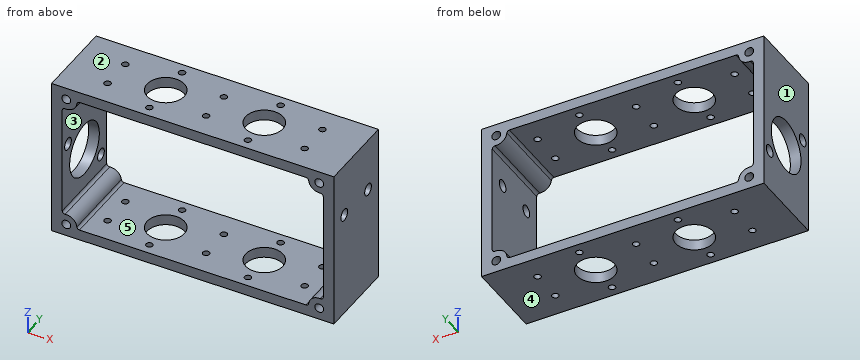
from build123d import *

# Parameters (mm, degrees)
SKETCH_1_W                                 = 106
SKETCH_1_H                                 = 60
EXTRUDE_1_DEPTH                            = 15
SKETCH_4_W                                 = 98
SKETCH_4_H                                 = 52
CUT_EXTRUDE_3_DEPTH                        = 68.88961629
SKETCH_5_R                                 = 2
EXTRUDE_2_DEPTH                            = 30
MIRROR_3_COPY_1_SKETCH_R                   = 2
MIRROR_3_COPY_1_DEPTH                      = 30
SKETCH_3_R                                 = 1.65
CUT_EXTRUDE_2_DEPTH                        = 10
CUT_EXTRUDE_4_REACH                        = 113.18
SKETCH_6_R                                 = 10
SKETCH_6_R_2                               = 2.25
SKETCH_7_R                                 = 2.25
CUT_EXTRUDE_5_DEPTH                        = 108.373181009
SKETCH_8_R                                 = 7
CUT_EXTRUDE_6_DEPTH                        = 82.449370777
HOLE_WIZARD_M3_1_D                         = 2.5
MIRROR_4_AT_THE_SECOND_PLANE_COPY_1_SKET_R = 7
MIRROR_4_AT_THE_SECOND_PLANE_COPY_1_DEPTH  = 82.449370777
MIRROR_4_AT_THE_SECOND_PLANE_COPY_2_D      = 2.5
EXTRUDE_START                              = -30
EXTRUDE_3_DEPTH                            = 30
FILLET_1_R                                 = 1


with BuildPart() as part:
    # 草图1 → 凸台-拉伸1 (new, symmetric)
    with BuildSketch(Plane(origin=(0, 0, 0), x_dir=(1, 0, 0), z_dir=(0, 1, 0))):
        Rectangle(SKETCH_1_W, SKETCH_1_H)
    extrude(amount=EXTRUDE_1_DEPTH, both=True)

    # 草图4 → 切除-拉伸3 (cut, through all)
    with BuildSketch(Plane(origin=(0, 15, 0), x_dir=(1, 0, 0), z_dir=(0, 1, 0))):
        Rectangle(SKETCH_4_W, SKETCH_4_H)
    extrude(amount=-CUT_EXTRUDE_3_DEPTH, mode=Mode.SUBTRACT)

    # 草图5 → 凸台-拉伸2 (add)
    with BuildSketch(Plane(origin=(0, 15, 0), x_dir=(1, 0, 0), z_dir=(0, 1, 0))):
        with Locations((47.5, 25.5)):
            Circle(SKETCH_5_R)
    extrude_2 = extrude(amount=-EXTRUDE_2_DEPTH)

    # 镜向2: 凸台-拉伸2 across plane
    add(extrude_2.mirror(Plane(origin=(0, 0, 0), x_dir=(0, 0, 1), z_dir=(1, 0, 0))))

    # 镜向3: 凸台-拉伸2 across plane
    add(extrude_2.mirror(Plane.XY))

    # 镜向3 copy 1 sketch → 镜向3 copy 1 (add)
    with BuildSketch(Plane(origin=(0, 15, 0), x_dir=(-1, 0, 0), z_dir=(0, 1, 0))):
        with Locations((47.5, 25.5)):
            Circle(MIRROR_3_COPY_1_SKETCH_R)
    extrude(amount=-MIRROR_3_COPY_1_DEPTH)

    # 草图3 → 切除-拉伸2 (cut)
    with BuildSketch(Plane(origin=(0, 15, 0), x_dir=(1, 0, 0), z_dir=(0, 1, 0))):
        with Locations(Location((47.5, 25.5, 0), (0, 0, 270))):
            Circle(SKETCH_3_R)
        with Locations(Location((47.5, -25.5, 0), (0, 0, 90))):
            Circle(SKETCH_3_R)
        with Locations(Location((-47.5, -25.5, 0), (0, 0, 270))):
            Circle(SKETCH_3_R)
        with Locations(Location((-47.5, 25.5, 0), (0, 0, 90))):
            Circle(SKETCH_3_R)
    cut_extrude_2 = extrude(amount=-CUT_EXTRUDE_2_DEPTH, mode=Mode.SUBTRACT)

    # 镜向1: 切除-拉伸2 across plane
    add(cut_extrude_2.mirror(Plane.ZX), mode=Mode.SUBTRACT)

    # 草图6 → 切除-拉伸4 (cut, up to next)
    with BuildSketch(Plane.ZY.offset(53), mode=Mode.PRIVATE) as cut_extrude_4_sk1:
        with Locations((-5, 0)):
            Circle(SKETCH_6_R)
    cut_extrude_4_tool1 = extrude(cut_extrude_4_sk1.sketch, amount=-CUT_EXTRUDE_4_REACH, mode=Mode.PRIVATE) & part.part
    # 草图6 → 切除-拉伸4 (cut, up to next)
    with BuildSketch(Plane.ZY.offset(53), mode=Mode.PRIVATE) as cut_extrude_4_sk2:
        with Locations((-14.32042034, 11.107644425)):
            Circle(SKETCH_6_R_2)
    cut_extrude_4_tool2 = extrude(cut_extrude_4_sk2.sketch, amount=-CUT_EXTRUDE_4_REACH, mode=Mode.PRIVATE) & part.part
    # 草图6 → 切除-拉伸4 (cut, up to next)
    with BuildSketch(Plane.ZY.offset(53), mode=Mode.PRIVATE) as cut_extrude_4_sk3:
        with Locations((4.32042034, -11.107644425)):
            Circle(SKETCH_6_R_2)
    cut_extrude_4_tool3 = extrude(cut_extrude_4_sk3.sketch, amount=-CUT_EXTRUDE_4_REACH, mode=Mode.PRIVATE) & part.part
    add(cut_extrude_4_tool1.solids().sort_by_distance((-53, 0, -5))[0], mode=Mode.SUBTRACT)
    add(cut_extrude_4_tool2.solids().sort_by_distance((-53, 11.107644, -14.32042))[0], mode=Mode.SUBTRACT)
    add(cut_extrude_4_tool3.solids().sort_by_distance((-53, -11.107644, 4.32042))[0], mode=Mode.SUBTRACT)

    # 草图7 → 切除-拉伸5 (cut, through all)
    with BuildSketch(Plane.ZY.offset(-49)):
        with Locations((10, 8)):
            Circle(SKETCH_7_R)
        with Locations((10, -8)):
            Circle(SKETCH_7_R)
    extrude(amount=-CUT_EXTRUDE_5_DEPTH, mode=Mode.SUBTRACT)

    # 草图8 → 切除-拉伸6 (cut, through all)
    with BuildSketch(Plane.XY.offset(30)):
        with Locations((18.5, 0)):
            Circle(SKETCH_8_R)
    cut_extrude_6 = extrude(amount=-CUT_EXTRUDE_6_DEPTH, mode=Mode.SUBTRACT)

    # M3 螺纹孔1 (through all)
    with Locations(Plane(origin=(0, 6, 30), x_dir=(1, 0, 0), z_dir=(0, 0, 1))):
        with Locations((0, 0), (18.5, 5), (37, 0)):
            hole_wizard_m3_1 = Hole(HOLE_WIZARD_M3_1_D / 2)

    # 镜向4: 切除-拉伸6, M3 螺纹孔1 across plane
    add(cut_extrude_6.mirror(Plane(origin=(0, 0, 0), x_dir=(0, 0, 1), z_dir=(1, 0, 0))), mode=Mode.SUBTRACT)
    add(hole_wizard_m3_1.mirror(Plane(origin=(0, 0, 0), x_dir=(0, 0, 1), z_dir=(1, 0, 0))), mode=Mode.SUBTRACT)

    # 镜向4 at the second plane: 切除-拉伸6, M3 螺纹孔1 across plane
    add(cut_extrude_6.mirror(Plane.ZX), mode=Mode.SUBTRACT)
    add(hole_wizard_m3_1.mirror(Plane.ZX), mode=Mode.SUBTRACT)

    # 镜向4 at the second plane copy 1 sket → 镜向4 at the second plane copy 1 (cut, through all)
    with BuildSketch(Plane(origin=(0, 0, 30), x_dir=(-1, 0, 0), z_dir=(0, 0, 1))):
        with Locations((18.5, 0)):
            Circle(MIRROR_4_AT_THE_SECOND_PLANE_COPY_1_SKET_R)
    extrude(amount=-MIRROR_4_AT_THE_SECOND_PLANE_COPY_1_DEPTH, mode=Mode.SUBTRACT)

    # 镜向4 at the second plane copy 2 (through all)
    with Locations(Plane(origin=(0, -6, 30), x_dir=(-1, 0, 0), z_dir=(0, 0, 1))):
        with Locations((0, 0), (18.5, 5), (37, 0)):
            Hole(MIRROR_4_AT_THE_SECOND_PLANE_COPY_2_D / 2)

    # 草图10 → 凸台-拉伸3 (add)
    with BuildSketch(Plane(origin=(0, 15, 0), x_dir=(1, 0, 0), z_dir=(0, 1, 0)).offset(EXTRUDE_START)):
        with BuildLine():
            ThreePointArc((-49, 21.791900756), (-45.06062414, 22.329913974), (-43.531373033, 26))
            Line((-43.531373033, 26), (-45.563508327, 26))
            ThreePointArc((-45.563508327, 26), (-46.562796629, 23.733180869), (-49, 24.177124344))
            Line((-49, 24.177124344), (-49, 21.791900756))
        make_face()
        with BuildLine():
            Line((45.563508327, 26), (43.531373033, 26))
            ThreePointArc((43.531373033, 26), (45.06062414, 22.329913974), (49, 21.791900756))
            Line((49, 21.791900756), (49, 24.177124344))
            ThreePointArc((49, 24.177124344), (46.562796629, 23.733180869), (45.563508327, 26))
        make_face()
        with BuildLine():
            ThreePointArc((-43.531373033, -26), (-45.06062414, -22.329913974), (-49, -21.791900756))
            Line((-49, -21.791900756), (-49, -24.177124344))
            ThreePointArc((-49, -24.177124344), (-46.562796629, -23.733180869), (-45.563508327, -26))
            Line((-45.563508327, -26), (-43.531373033, -26))
        make_face()
        with BuildLine():
            Line((49, -24.177124344), (49, -21.791900756))
            ThreePointArc((49, -21.791900756), (45.06062414, -22.329913974), (43.531373033, -26))
            Line((43.531373033, -26), (45.563508327, -26))
            ThreePointArc((45.563508327, -26), (46.562796629, -23.733180869), (49, -24.177124344))
        make_face()
    extrude(amount=EXTRUDE_3_DEPTH)

    # 圆角1
    fillet_1_edges = [part.edges().sort_by_distance(p)[0] for p in [
        (49, 0, -21.791900756),
        (43.531373033, 0, -26),
        (43.531373033, 0, 26),
        (49, 0, 21.791900756),
        (-49, 0, 21.791900756),
        (-43.531373033, 0, 26),
        (-43.531373033, 0, -26),
        (-49, 0, -21.791900756),
    ]]
    fillet(fillet_1_edges, radius=FILLET_1_R)


solid = part.part
Source: CAD feature listing. Evaluate the final solid. Frame: model axes, mm. Face numbers are marked on the shaded views. A direction names the side the tool comes from. Give positions to 0.01 mm unless a question says otherwise; leave off trailing zeros. Write each loop counter-clockwise with the first axis right and the second up, starting at its lowest first coordinate (ties: lowest second). Pieces come first, ordered by that corner, then holes. Notation, with made-up numbers: (0, 52) - (22, 52) arc R20 ccw to (22, 85) - close; hole circle Ø3 at (-29, 1.25). An arc over 180 degrees is marked (long way). Write item = value, one per line. Start each with the question number.
Q1. Cut plane A-A, the plane x = 8. Return loops of the section in (y, z), then the cut area to 3 significant figures.
Q2. Draft query along X for the marked faces 1, 2 and 3. Return one class per face: +X half, -X half, draft (parallel to the pull), parting line (faces both ways), or undercut.
Q3. Pin query (flat end, axial travel): pin 1 Ø5 at (y, z) = (0.5, 1) entering from -X; pin 2 Ø2 at (x, z) = (-47.5, 25.5) entering from -Y. Return the tip coordinate at first contact, or that it passes through.
Q4. Material intervals for probe 1 along Y at (x, z) = (0, -28.35); probe 2 along Y at (x, z) = (-18.5, -28.4); probe 3 along Y at (x, z) = (51.25, 10), sorted ascending.
Q5. Cut plane B-B, the plane z = 15. Return loops of the section in (x, y).
Q6. Cut plane D-D, the plane x = -23. Return loops of the section in (y, z), then the cut area to 3 significant figures.
Q7. Reachability of the marked faces 4 and 5 from +Z, -Z, +X, -X, +Y, -Y: full face, straight path, thin tool, end or side. Return the list, or none.
Q8. Cut plane C-C, the plane x = -37. Return loops of the section in (y, z), then the cut area to 3 significant figures.
Computed values:
q1.outline = (-15, -30) - (15, -30) - (15, -26) - (-15, -26) - close; (-15, 26) - (15, 26) - (15, 30) - (-15, 30) - close
q1.area = 240 mm²
q2.face_1 = -X half
q2.face_2 = draft
q2.face_3 = undercut
q3.pin_1 = 49
q3.pin_2 = -5
q4.probe_1 = -15 to -7.25, -4.75 to 4.75, 7.25 to 15
q4.probe_2 = -15 to -12.25, -9.75 to -7, 7 to 9.75, 12.25 to 15
q4.probe_3 = -15 to -10.25, -5.75 to 5.75, 10.25 to 15
q5.outline = (-53, -15) - (-49, -15) - (-49, 15) - (-53, 15) - close; (49, -15) - (53, -15) - (53, 15) - (49, 15) - close
q6.outline = (-15, -30) - (-5.36, -30) - (-5.36, -26) - (-15, -26) - close; (-15, 26) - (-5.36, 26) - (-5.36, 30) - (-15, 30) - close; (5.36, -30) - (15, -30) - (15, -26) - (5.36, -26) - close; (5.36, 26) - (15, 26) - (15, 30) - (5.36, 30) - close
q6.area = 154 mm²
q7.face_4 = -Z, +X, -X, +Y, -Y
q7.face_5 = +Y, -Y
q8.outline = (-15, -30) - (-7.25, -30) - (-7.25, -26) - (-15, -26) - close; (-15, 26) - (-7.25, 26) - (-7.25, 30) - (-15, 30) - close; (-4.75, -30) - (4.75, -30) - (4.75, -26) - (-4.75, -26) - close; (-4.75, 26) - (4.75, 26) - (4.75, 30) - (-4.75, 30) - close; (7.25, -30) - (15, -30) - (15, -26) - (7.25, -26) - close; (7.25, 26) - (15, 26) - (15, 30) - (7.25, 30) - close
q8.area = 200 mm²
